```python
from build123d import *

# Parameters (mm, degrees)
SKETCH_1_R          = 50
EXTRUDE_1_DEPTH     = 20
CUT_EXTRUDE_1_DEPTH = 17
SKETCH_3_R          = 7.9
SKETCH_3_R_2        = 4
EXTRUDE_2_DEPTH     = 4
CUT_EXTRUDE_2_DEPTH = 5
SKETCH_7_R          = 1.8
CUT_EXTRUDE_3_DEPTH = 19
SKETCH_8_W          = 40
SKETCH_8_H          = 17
CUT_EXTRUDE_4_DEPTH = 2
FILLET_1_R          = 10
SKETCH_10_R         = 2.5
CUT_EXTRUDE_5_DEPTH = 10
SKETCH_11_R         = 1.5
CUT_EXTRUDE_6_DEPTH = 10


with BuildPart() as part:
    # 草图1 → 凸台-拉伸1 (new body)
    with BuildSketch(Plane.XY):
        Circle(SKETCH_1_R)
    extrude(amount=EXTRUDE_1_DEPTH)

    # 草图2 → 切除-拉伸1 (cut)
    with BuildSketch(Plane.XY.offset(20)):
        Polygon((-20, -37), (-20, 0), (-20, 40), (20, 40), (20, -58.754478709), (-20, -58.754478709), align=None)
    extrude(amount=-CUT_EXTRUDE_1_DEPTH, mode=Mode.SUBTRACT)

    # 草图3 → 凸台-拉伸2 (add)
    with BuildSketch(Plane.XY.offset(3)):
        with Locations((0, -39)):
            Circle(SKETCH_3_R)
        with Locations((0, -39)):
            Circle(SKETCH_3_R_2, mode=Mode.SUBTRACT)
    extrude(amount=EXTRUDE_2_DEPTH)

    # 草图5 → 切除-拉伸2 (cut)
    with BuildSketch(Plane.XY.offset(20)):
        Polygon((37.5, -20), (33.5, -20), (33.5, 20), (41.5, 20), (41.5, -20), align=None)
    cut_extrude_2 = extrude(amount=-CUT_EXTRUDE_2_DEPTH, mode=Mode.SUBTRACT)

    # 草图7 → 切除-拉伸3 (cut)
    with BuildSketch(Plane(origin=(0, -20, 0), x_dir=(1, 0, 0), z_dir=(0, 1, 0))):
        with Locations((37.5, -20)):
            Circle(SKETCH_7_R)
    cut_extrude_3 = extrude(amount=-CUT_EXTRUDE_3_DEPTH, mode=Mode.SUBTRACT)

    # 镜向1: 切除-拉伸2, 切除-拉伸3 across plane
    add(cut_extrude_2.mirror(Plane(origin=(0, 0, 0), x_dir=(0, 0, 1), z_dir=(1, 0, 0))), mode=Mode.SUBTRACT)
    add(cut_extrude_3.mirror(Plane(origin=(0, 0, 0), x_dir=(0, 0, 1), z_dir=(1, 0, 0))), mode=Mode.SUBTRACT)

    # 草图8 → 切除-拉伸4 (cut)
    with BuildSketch(Plane.XZ.offset(-40)):
        with Locations((0, 11.5)):
            Rectangle(SKETCH_8_W, SKETCH_8_H)
    extrude(amount=-CUT_EXTRUDE_4_DEPTH, mode=Mode.SUBTRACT)

    # 圆角1
    # the kernel refuses this fillet: 10 mm, written as the material it takes off along each edge
    with BuildSketch(Plane(origin=(0, 0, 0), x_dir=(1, 0, 0), z_dir=(0, -1, 0))) as fillet_1_piece_1:
        with BuildLine():
            CenterArc((50 - FILLET_1_R, FILLET_1_R), FILLET_1_R, 270, 90)
            Line((50 - FILLET_1_R, 0), (50, 0))
            Line((50, 0), (50, FILLET_1_R))
        make_face()
    revolve(axis=Axis((0, 0, 0), (0, 0, 1)), mode=Mode.SUBTRACT)

    # 草图10 → 切除-拉伸5 (cut)
    with BuildSketch(Plane(origin=(0, 0, 0), x_dir=(-1, 0, 0), z_dir=(0, 0, -1))):
        with Locations((25, 0)):
            Circle(SKETCH_10_R)
        with Locations((-25, 0)):
            Circle(SKETCH_10_R)
    extrude(amount=-CUT_EXTRUDE_5_DEPTH, mode=Mode.SUBTRACT)

    # 草图11 → 切除-拉伸6 (cut)
    with BuildSketch(Plane(origin=(0, 0, 10), x_dir=(-1, 0, 0), z_dir=(0, 0, -1))):
        with Locations((-25, 0)):
            Circle(SKETCH_11_R)
        with Locations((25, 0)):
            Circle(SKETCH_11_R)
    extrude(amount=-CUT_EXTRUDE_6_DEPTH, mode=Mode.SUBTRACT)


solid = part.part
```
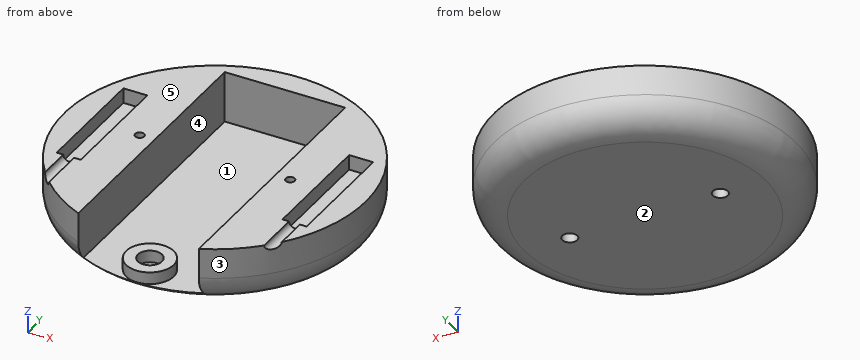
Here's how the part is built. I have some questions about the finished solid (model axes, mm). Face numbers are marked on the shaded views. A direction names the side the tool comes from. Round coordinates to 2 decimals unless told otherwise and drop trailing zeros. One line per question, with ' | ' between items.
1) I need wall thicknesses on line 1 along X through (y, z) = (-11, 18.25) (3 decimals); line 2 along X through (y, z) = (6, 19); line 3 along X through (y, z) = (11.5, 7.75). Which ranges of each line are inside material? Lowest first, please.
Working result:
line 1: -48.775 to -41.5, -33.5 to -20, 20 to 33.5, 41.5 to 48.775 | line 2: -49.64 to -41.5, -33.5 to -20, 20 to 33.5, 41.5 to 49.64 | line 3: -48.4 to -20, 20 to 48.4
2) For pin 1 Ø5.5 at (x, z) = (-38, 17) entering from -Y; pin 2 Ø2.5 at (x, y) = (25.5, -1) entering from -Z; pin 3 Ø2 at (x, z) = (-7, 16) entering from -Y; pin 4 Ø2.5 at (x, y) = (-25, 0) entering from -Z, each with a flat end and sliding along its axis, tell me the tip position at first contact or that it passes through.
Working result:
pin 1: y = -35.46 | pin 2: z = 10 | pin 3: y = 42 | pin 4: through
3) If we mould it in two halves opening along Y, with no side actions, what happens to the marked faces 1, 2 and 3? For each: +Y half, -Y half, draft (parallel to the pull), parting line (faces both ways), or undercut.
Working result:
face 1: undercut | face 2: draft | face 3: parting line
4) I want a section at A-A, the plane y = 0. State how many separate pieces and enclosed holes the cut face has, then the cut area to 3 significant figures.
Working result:
separate pieces: 3 | enclosed holes: 0 | area: 1,040 mm²
5) For the marked faces 4 and 5, which set-ups out of +Z, -Z, +X, -X, +Y, -Y let a thin tool reach every point of the face, with its end or its side?
Working result:
face 4: +Z, -Y | face 5: +Z, +X, -X, +Y, -Y
